Input: part model. Units: mm. Frame: model coordinates. A direction names the side the tool comes from. Coordinates: 2 decimals unless noted, no trailing zeros. Loops run counter-clockwise (first coordinate to the right, second up) from the corner with the lowest first, then second, coordinate; pieces in that order, holes last.
(1) Line query: L1, parallel to Z at x = 0, y = 28.25; L2, parallel to X at y = -19, z = 5; L3, parallel to X at y = 35.25, z = 10. Output: solid intervals per line, ascending.
(2) Section C-C, the plane y = 22. Return loops of the section in (x, z).
(3) Mould query, pull axis Y, two halves, no side actions, for faces 5 (the face through (32, -36, 10)), 6 (the face through (30, -12, 10)), 7 (the face through (-12, 39, 10)), 8 (the face through (-27, -23.817, 10)). Classes: released by +Y, released by -Y, zero draft, split by the parting line, or undercut.
(4) Section D-D, the plane z = 3.75. Return loops of the section in (x, y).
(5) Section B-B, the plane z = 10. Return loops of the section in (x, y), then the cut area to 3 significant figures.
(6) Section A-A, the plane x = 0. Return loops of the section in (y, z).
(7) Set-up query: faces 1 (the face through (-29.251, 20.985, 9.86)), 2 (the face through (-27, 0, 10)), 3 (the face through (12, 39, 10)), 4 (the face through (-24, -30, 10)). Return all of +Z, -Z, +X, -X, +Y, -Y with unobstructed straight access to the full face (end or side cutting, diameter ignored); none if empty.
(8) Contact query for flat-ended pins moving along their axis: P1, Ø2, axis at y = 17, z = 7, coming from the -X side; P2, Ø8, axis at x = -31.5, z = 7.5, coming from the +Y side; P3, Ø2.5, axis at y = 39, z = 5.5, coming from the +X side. Output: stop coordinate, or through.
```python
from build123d import *

# Parameters (mm, degrees)
Y_KSEKLIK_EKSTR_ZYON1_DEPTH = 20
IZIM2_R                     = 5.251294355
KES_EKSTR_ZYON1_DEPTH       = 35


with BuildPart() as part:
    # Çizim1 → Yükseklik-Ekstrüzyon1 (new body)
    with BuildSketch(Plane.XY):
        with BuildLine():
            Line((39.799497484, 0), (40, 0))
            Line((40, 0), (40, -36))
            Line((40, -36), (24, -36))
            Line((24, -36), (24, -23.81673939))
            Line((24, -23.81673939), (30, -23.81673939))
            Line((30, -23.81673939), (30, 0))
            Line((30, 0), (24, 0))
            ThreePointArc((24, 0), (0, 24), (-24, 0))
            Line((-24, 0), (-30, 0))
            Line((-30, 0), (-30, -23.81673939))
            Line((-30, -23.81673939), (-24, -23.81673939))
            Line((-24, -23.81673939), (-24, -36))
            Line((-24, -36), (-40, -36))
            Line((-40, -36), (-40, 0))
            Line((-40, 0), (-39.799497484, 0))
            ThreePointArc((-39.799497484, 0), (-37.116215911, 1.033520605), (-35.819547736, 3.6))
            ThreePointArc((-35.819547736, 3.6), (-29.094854574, 21.201165942), (-14.4, 32.994545004))
            ThreePointArc((-14.4, 32.994545004), (-12.653359894, 34.46971533), (-12, 36.66060556))
            Line((-12, 36.66060556), (-12, 41.66060556))
            Line((-12, 41.66060556), (12, 41.66060556))
            Line((12, 41.66060556), (12, 36.66060556))
            ThreePointArc((12, 36.66060556), (12.653359894, 34.46971533), (14.4, 32.994545004))
            ThreePointArc((14.4, 32.994545004), (29.094854574, 21.201165942), (35.819547736, 3.6))
            ThreePointArc((35.819547736, 3.6), (37.116215911, 1.033520605), (39.799497484, 0))
        make_face()
    extrude(amount=Y_KSEKLIK_EKSTR_ZYON1_DEPTH)

    # Çizim2 → Kes-Ekstrüzyon1 (cut)
    with BuildSketch(Plane(origin=(0, 41.66060556, 0), x_dir=(1, 0, 0), z_dir=(0, 1, 0))):
        with Locations((0, -10)):
            Circle(IZIM2_R)
    extrude(amount=-KES_EKSTR_ZYON1_DEPTH, mode=Mode.SUBTRACT)


solid = part.part
```
Report:
1. L1: z = 0 to 4.75, 15.25 to 20
1. L2: x = -40 to -30, 30 to 40
1. L3: x = -12.26 to -5.25, 5.25 to 12.26
2. outline: (-28.5, 0) - (-9.59, 0) - (-9.59, 20) - (-28.5, 20) - close; (9.59, 0) - (28.5, 0) - (28.5, 20) - (9.59, 20) - close
3. face 5: released by -Y
3. face 6: undercut
3. face 7: zero draft
3. face 8: undercut
4. outline: (-40, -36) - (-24, -36) - (-24, -23.82) - (-30, -23.82) - (-30, 0) - (-24, 0) arc R24 cw to (24, 0) - (30, 0) - (30, -23.82) - (24, -23.82) - (24, -36) - (40, -36) - (40, 0) - (39.8, 0) arc R4 cw to (35.82, 3.6) arc R36 ccw to (14.4, 32.99) arc R4 cw to (12, 36.66) - (12, 41.66) - (-12, 41.66) - (-12, 36.66) arc R4 cw to (-14.4, 32.99) arc R36 ccw to (-35.82, 3.6) arc R4 cw to (-39.8, 0) - (-40, 0) - close
5. outline: (-40, -36) - (-24, -36) - (-24, -23.82) - (-30, -23.82) - (-30, 0) - (-24, 0) arc R24 cw to (-5.25, 23.42) - (-5.25, 41.66) - (-12, 41.66) - (-12, 36.66) arc R4 cw to (-14.4, 32.99) arc R36 ccw to (-35.82, 3.6) arc R4 cw to (-39.8, 0) - (-40, 0) - close; (5.25, 23.42) arc R24 cw to (24, 0) - (30, 0) - (30, -23.82) - (24, -23.82) - (24, -36) - (40, -36) - (40, 0) - (39.8, 0) arc R4 cw to (35.82, 3.6) arc R36 ccw to (14.4, 32.99) arc R4 cw to (12, 36.66) - (12, 41.66) - (5.25, 41.66) - close
5. area: 1,970 mm2
6. outline: (24, 0) - (41.66, 0) - (41.66, 4.75) - (24, 4.75) - close; (24, 15.25) - (41.66, 15.25) - (41.66, 20) - (24, 20) - close
7. face 1: +Z, -Z, -X, +Y
7. face 2: +Z, -Z
7. face 3: +Z, -Z, +X, +Y
7. face 4: +Z, -Z, -Y
8. P1: stops at x = -32.25
8. P2: stops at y = 23.23
8. P3: stops at x = 12
